```python
from build123d import *

# Parameters (mm, degrees)
F2_W           = 8.5
F2_H           = 9.2348072443
F3_DEPTH       = 22
F5_D           = 8
F5_DEPTH       = 20
F5_TIP         = 2.4034424761
F6_R           = 0.5
F8_D           = 5
F8_DEPTH       = 12
F8_CSINK_D     = 7
F8_CSINK_ANGLE = 60
F8_TIP         = 1.5021515476


with BuildPart() as f1:
    # F0 (on Front) → F1 (revolve)
    with BuildSketch(Plane.XZ):
        Polygon((-21, 6.5), (-21, 0), (87.5, 0), (87.5, 7.5), (0, 7.5), (0, 11), (-4, 11), (-4, 7.5397645426), align=None)
    revolve(axis=Axis((33.25, 0, 0), (1, 0, 0)))

    # F2 (on face) → F3 (join)
    with BuildSketch(Plane.YZ.offset(87.5)):
        Rectangle(F2_W, F2_H)
    extrude(amount=F3_DEPTH)

    # F5
    with Locations(Plane(origin=(-21, 0, 0), x_dir=(0, -1, 0), z_dir=(-1, 0, 0))):
        with Locations((0, 0)):
            Hole(F5_D / 2, depth=F5_DEPTH)
            with Locations((0, 0, -(F5_DEPTH + F5_TIP / 2))):  # 118° drill point
                Cone(0, F5_D / 2, F5_TIP, mode=Mode.SUBTRACT)

    # F6
    f6_edges = [f1.edges().sort_by_distance(p)[0] for p in [
        (98.5, -4.25, 4.617404),
        (98.5, -4.25, -4.617404),
        (98.5, 4.25, 4.617404),
        (98.5, 4.25, -4.617404),
    ]]
    fillet(f6_edges, radius=F6_R)

    # F8
    with Locations(Plane.YZ.offset(109.5)):
        with Locations((0, 0)):
            CounterSinkHole(F8_D / 2, F8_CSINK_D / 2, depth=F8_DEPTH, counter_sink_angle=F8_CSINK_ANGLE)
            with Locations((0, 0, -(F8_DEPTH + F8_TIP / 2))):  # 118° drill point
                Cone(0, F8_D / 2, F8_TIP, mode=Mode.SUBTRACT)


solid = f1.part
```
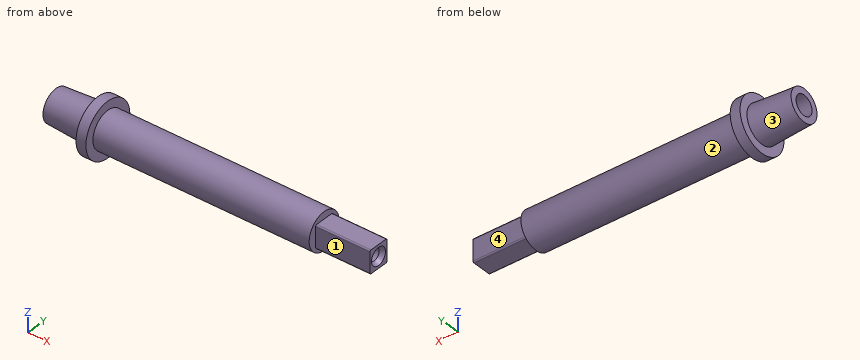
Can you work these out from the model? Positions are in its coordinate system, mm. Face numbers are marked on the shaded views. A direction names the side the tool comes from. Coordinates: 2 decimals unless noted, no trailing zeros. Loops run counter-clockwise (first coordinate to the right, second up) from the corner with the lowest first, then second, coordinate; pieces in that order, holes last.
1) I need wall thicknesses on probe 1 along Z at (x, y) = (100, 0); probe 2 along Y at (x, z) = (101.5, 0); probe 3 along Z at (x, y) = (32, 0). Which ranges of each line are inside material? Lowest first, please.
2) Which directions (+Z, -Z, +X, -X, +Y, -Y) give clear straight access to the entire face, cutting with the end or side of a thin tool? Please do the marked faces 1, 2, 3 and 4.
3) Imagine slicing it at C-C on y = -9.5. List the corners of the cut face in (x, z) for me, plus the area to 3 significant figures.
4) Imagine slicing it at D-D on x = 46. List the corners of the cut face in (y, z) for me, plus the area to 3 significant figures.
5) Imagine slicing it at A-A on x = 91.5. List the corners of the cut face in (y, z) for me.
6) For pin 1 (4 mm diameter, centred on x = 96.5, y = -0.5, fed in from +Z); pin 2 (10 mm diameter, centred on x = 46, y = 6, fed in from +Z); pin 3 (8 mm diameter, centred on y = 0, z = 0, fed in from +X); pin 4 (10 mm diameter, centred on x = 84, y = -4, fed in from +Z), each with a flat end and sliding along its axis, tell me the tip position at first contact or that it passes through.
7) Imagine slicing it at B-B on x = -6. List the corners of the cut face in (y, z) for me.
Completed:
1. probe 1: z = -4.62 to -2.5, 2.5 to 4.62
1. probe 2: y = -4.25 to -2.5, 2.5 to 4.25
1. probe 3: z = -7.5 to 7.5
2. face 1: +Z, -Z, +X, -Y
2. face 2: +X
2. face 3: -X
2. face 4: +Z, -Z, +X, +Y
3. outline: (-4, -5.55) - (0, -5.55) - (0, 5.55) - (-4, 5.55) - close
3. area: 44.4 mm2
4. outline: circle Ø15 at (0, 0)
4. area: 177 mm2
5. outline: (-4.25, -4.12) arc R0.5 ccw to (-3.75, -4.62) - (3.75, -4.62) arc R0.5 ccw to (4.25, -4.12) - (4.25, 4.12) arc R0.5 ccw to (3.75, 4.62) - (-3.75, 4.62) arc R0.5 ccw to (-4.25, 4.12) - close
6. pin 1: stops at z = 4.62
6. pin 2: stops at z = 7.43
6. pin 3: stops at x = 109.5
6. pin 4: stops at z = 7.5
7. outline: circle Ø14.83 at (0, 0); hole circle Ø8 at (0, 0)
